The figure shows three views and two pictorial views of one solid part (mm, origin at its lowest corner). Answer the questions. A direction names the side the tool comes from. Give positions to 0.01 mm unless a question says otherwise; leave off trailing zeros. Loops run counter-clockwise (first coordinate to the right, second up) from the corner with the lowest first, then second, coordinate; pieces in that order, holes last.
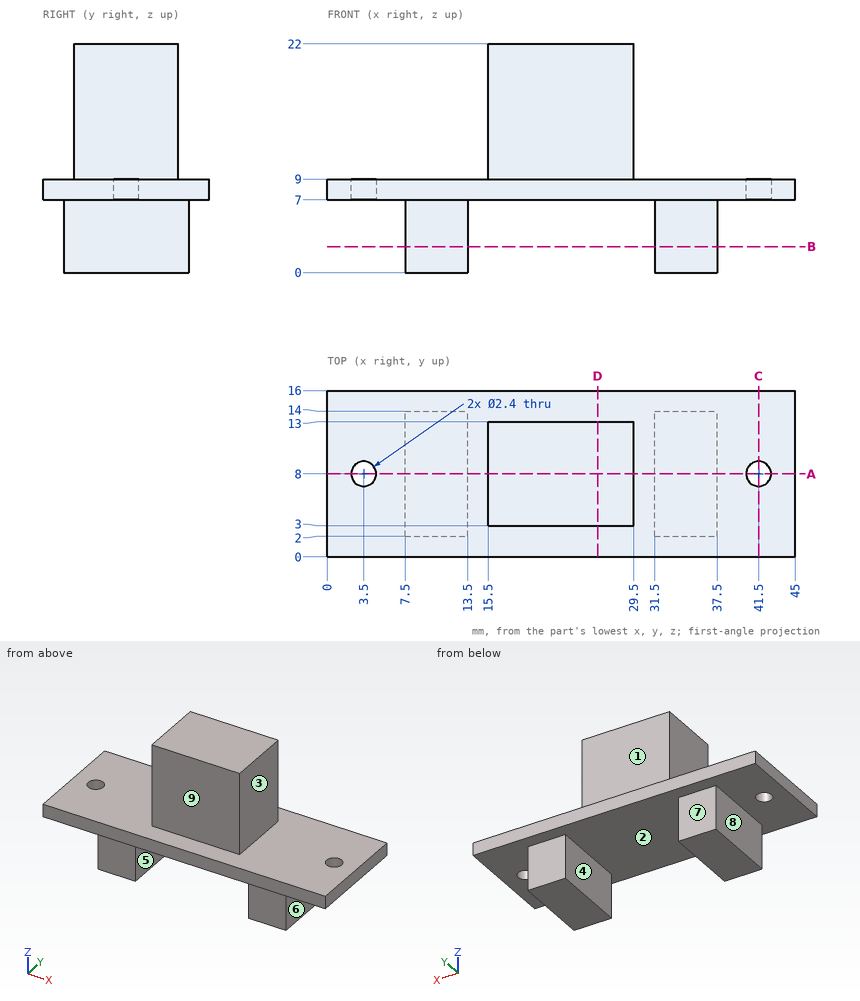
Q1. Section A-A on y = 8 is taken. Give the vertices of the cut face in (x, z), plus the area to 3 significant figures.
Q2. Section C-C on x = 41.5 is taken. Give the vertices of the cut face in (y, z).
Q3. Which of the six approach directions +Z, -Z, +X, -X, +Y, -Y give full straight-line access (tool end or side, diameter ignored) to the marked faces 5, 6, 7, 8 and 9?
Q4. Consider line 1 along Y through (x, z) = (3.5, 8.2); line 2 along X through (y, z) = (7.75, 5.75); line 3 along Z through (x, y) = (15, 13.25). Determine where each line is inside the solid, lowest interval first.
Q5. Section D-D on x = 26 is taken. Give the vertices of the cut face in (y, z).
Q6. Given pin 1 (3.5 mm diameter, centred on y = 6, z = 2.5, fed in from +X); pin 2 (8 mm diameter, centred on y = 9, z = 17, fed in from -X); pin 3 (2 mm diameter, centred on y = 8.5, z = 2.5, fed in from -X), each flat-ended and moving along its own axis, determine where each tip first touches the part or whether it passes through.
Q7. Section B-B on z = 2.5 is taken. Give the vertices of the cut face in (x, y).
Q8. Determine the mould class of the marked faces 1, 2, 3 and 4 for opening direction X: +X half, -X half, draft (parallel to the pull), parting line (faces both ways), or undercut.
Check result:
1. outline: (0, 7) - (2.3, 7) - (2.3, 9) - (0, 9) - close; (4.7, 7) - (7.5, 7) - (7.5, 0) - (13.5, 0) - (13.5, 7) - (31.5, 7) - (31.5, 0) - (37.5, 0) - (37.5, 7) - (40.3, 7) - (40.3, 9) - (29.5, 9) - (29.5, 22) - (15.5, 22) - (15.5, 9) - (4.7, 9) - close; (42.7, 7) - (45, 7) - (45, 9) - (42.7, 9) - close
1. area: 346 mm2
2. outline: (0, 7) - (6.8, 7) - (6.8, 9) - (0, 9) - close; (9.2, 7) - (16, 7) - (16, 9) - (9.2, 9) - close
3. face 5: -Z, +Y, -Y
3. face 6: -Z, +X, +Y, -Y
3. face 7: -Z, +X, -X, +Y
3. face 8: -Z, -X, +Y, -Y
3. face 9: +Z, +X, -X, -Y
4. line 1: y = 0 to 6.8, 9.2 to 16
4. line 2: x = 7.5 to 13.5, 31.5 to 37.5
4. line 3: z = 7 to 9
5. outline: (0, 7) - (16, 7) - (16, 9) - (13, 9) - (13, 22) - (3, 22) - (3, 9) - (0, 9) - close
6. pin 1: stops at x = 37.5
6. pin 2: stops at x = 15.5
6. pin 3: stops at x = 7.5
7. outline: (7.5, 2) - (13.5, 2) - (13.5, 14) - (7.5, 14) - close; (31.5, 2) - (37.5, 2) - (37.5, 14) - (31.5, 14) - close
8. face 1: draft
8. face 2: undercut
8. face 3: +X half
8. face 4: undercut
